from build123d import *

# Parameters (mm, degrees)
SFAZOWANIE1_SIZE = 0.5


with BuildPart() as part:
    # Szkic1 → Obrót1 (revolve)
    with BuildSketch(Plane.XY):
        with BuildLine():
            Line((-6, 0), (6, 0))
            Line((6, 0), (6, 1.2))
            ThreePointArc((6, 1.2), (5.282017059, 1.822044839), (4.5, 2.361385739))
            Line((4.5, 2.361385739), (4.5, 5.5))
            Line((4.5, 5.5), (-4.5, 5.5))
            Line((-4.5, 5.5), (-4.5, 2.361385739))
            ThreePointArc((-4.5, 2.361385739), (-5.282017059, 1.822044839), (-6, 1.2))
            Line((-6, 1.2), (-6, 0))
        make_face()
    revolve(axis=Axis((-11.261323988, -4, 0), (1, 0, 0)))

    # Sfazowanie1
    sfazowanie1_edges = [part.edges().sort_by_distance(p)[0] for p in [
        (-4.5, -13.5, 0),
        (4.5, -13.5, 0),
    ]]
    chamfer(sfazowanie1_edges, length=SFAZOWANIE1_SIZE)


solid = part.part
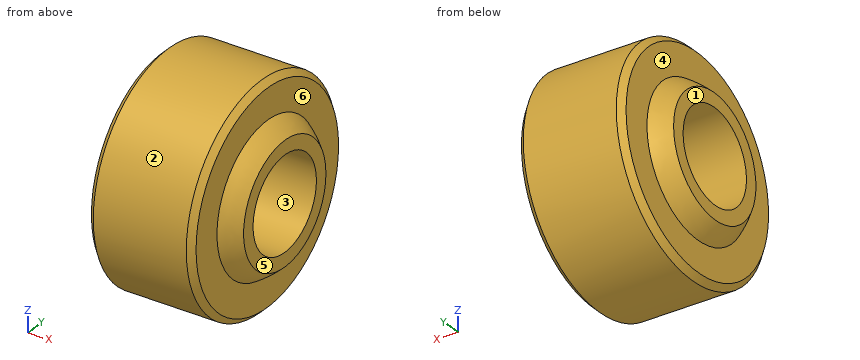
Input: part model. Units: mm. Frame: model coordinates. Face numbers are marked on the shaded views. A direction names the side the tool comes from. Coordinates: 2 decimals unless noted, no trailing zeros. Loops run counter-clockwise (first coordinate to the right, second up) from the corner with the lowest first, then second, coordinate; pieces in that order, holes last. Notation, with made-up numbers: (11.25, 8.25) -> (32.25, 8.25) arc R14 cw to (32.25, 26.25) -> close; hole circle Ø11 at (84.25, -9). An arc over 180 degrees is marked (long way). Write item = value, one per line. Start each with the question number.
Item 1: Cut plane A-A, the plane x = 0.5. Return loops of the section in (y, z).
Item 2: Material intervals for line 1 (Z direction, x = 1, y = -4); line 2 (X direction, y = -4, z = 7); line 3 (Y direction, x = -3.75, z = 2.75), sorted ascending.
Item 3: Reachability of the marked faces 4, 5 and 6 from +Z, -Z, +X, -X, +Y, -Y: full face, straight path, thin tool, end or side. Return the list, or none.
Item 4: First-contact query: P1, Ø5, axis at x = -1, y = -10.5, coming from the +Z side; P2, Ø1.5, axis at y = -1.5, z = -1.5, coming from the -X side; P3, Ø6, axis at y = 3.5, z = 7.5, coming from the +X side; P4, Ø8, axis at y = -11, z = -7, coming from the +X side. Flat tips, straight axial feed; report the tip coordinate or a pass-through.
Item 5: Mould query, pull axis Z, two halves, no side actions, for the marked faces 1, 2 and 3. Classes: pulls with the +Z half, pulls with the -Z half, needs draft (parallel to the pull), parting line crosses it, or undercut.
Ans:
q1.outline = circle Ø19 at (-4, 0); hole circle Ø8 at (-4, 0)
q2.line_1 = -9.5 to -4, 4 to 9.5
q2.line_2 = -4.5 to 4.5
q2.line_3 = -13.09 to -6.9, -1.1 to 5.09
q3.face_4 = -X
q3.face_5 = +Z, -Z, +X, +Y, -Y
q3.face_6 = +X
q4.P1 = 8.62
q4.P2 = through
q4.P3 = 4.5
q4.P4 = 5.18
q5.face_1 = needs draft
q5.face_2 = parting line crosses it
q5.face_3 = undercut
